Autodesk Inventor part; units mm, degrees
ref_plane "YZ Plane" through (0, 0, 0) normal (1, 0, 0) x (0, 1, 0)
ref_plane "XZ Plane" through (0, 0, 0) normal (0, 1, 0) x (-1, 0, 0)
ref_plane "XY Plane" through (0, 0, 0) normal (0, 0, 1) x (1, 0, 0)
sketch "Sketch2" plane through (0, 0, 0) normal (0, 0, 1) x (1, 0, 0)
  line L0 (-20, -20) -> (20, -20)
  line L1 (20, -20) -> (20, 20)
  line L2 (20, 20) -> (-20, 20)
  line L3 (-20, 20) -> (-20, -20)
  line L4 (-20, -20) -> (20, 20) construction
  line L5 (20, -20) -> (-20, 20) construction
  line L6 (-10, -10) -> (10, -10) construction
  line L7 (10, -10) -> (10, 10) construction
  line L8 (10, 10) -> (-10, 10) construction
  line L9 (-10, 10) -> (-10, -10) construction
  line L10 (-10, -10) -> (10, 10) construction
  line L11 (10, -10) -> (-10, 10) construction
  point P0 (0, 0)
  dimension "d0" = 40
  dimension "d1" = 40
  dimension "d2" = 20
  dimension "d3" = 20
extrude "Extrusion1" add sketch "Sketch2" along normal blind 5
hole "Hole1" at (-10, 10, 0) at (10, 10, 0) at (10, -10, 0) at (-10, -10, 0) direction (0, 0, 1) diameter 5.5 end through all
fillet "Fillet1" radius 2 4 edges at (20, 20, 2.5) (-20, 20, 2.5) (-20, -20, 2.5) (20, -20, 2.5)
properties part number "4040Square"
Input: part model. Units: mm. Frame: model coordinates. Give positions to 0.01 mm unless a question says otherwise; leave off trailing zeros. Loops run counter-clockwise (first coordinate to the right, second up) from the corner with the lowest first, then second, coordinate; pieces in that order, holes last. Notation, with made-up numbers: (55.5, 12) -> (94.5, 12) arc R23 cw to (94.5, 30) -> close; hole circle Ø11 at (-29.5, -19). An arc over 180 degrees is marked (long way). Use a Markdown table: item, result.
Q1. Pull-direction query (X, two-part tool) for faces 1 (the flat face through (0, 0, 5)), 2 (the cylindrical face through (-19.43, -19.4, 2.54)), 3 (the cylindrical face through (11.05, -7.46, 2.54)), 4 (the cylindrical face through (19.43, 19.4, 2.54)); classes: pulls with the +X half, pulls with the -X half, needs draft (parallel to the pull), parting line crosses it, or undercut.
Entries:
| item | result |
|---|---|
| face 1 | needs draft |
| face 2 | pulls with the -X half |
| face 3 | undercut |
| face 4 | pulls with the +X half |
Q2. Ray query, probe 1 along Y at (x, z) = (-10, 1.35); probe 2 along Y at (x, z) = (-11, 3.7); probe 3 along X at (y, z) = (8.5, 0.85). Return the intervals inside material, ascending. Write a range as from..to.
Entries:
| item | result |
|---|---|
| probe 1 | y = -20..-12.75, -7.25..7.25, 12.75..20 |
| probe 2 | y = -20..-12.56, -7.44..7.44, 12.56..20 |
| probe 3 | x = -20..-12.3, -7.7..7.7, 12.3..20 |
Q3. Section query A-A, the plane x = 10. Return the cut outline in (y, z).
Entries:
| item | result |
|---|---|
| outline | (-20, 0) -> (-12.75, 0) -> (-12.75, 5) -> (-20, 5) -> close; (-7.25, 0) -> (7.25, 0) -> (7.25, 5) -> (-7.25, 5) -> close; (12.75, 0) -> (20, 0) -> (20, 5) -> (12.75, 5) -> close |
Q4. First-contact query: P1, Ø5, axis at x = 10, y = 10, coming from the +Z side. Flat tip, straight axial feed; report the tip coordinate or a pass-through.
Entries:
| item | result |
|---|---|
| P1 | passes through |
Q5. Section query C-C, the plane z = 2.75. Return the cut outline in (x, y), plus the area to 3 significant figures.
Entries:
| item | result |
|---|---|
| outline | (-20, -18) arc R2 ccw to (-18, -20) -> (18, -20) arc R2 ccw to (20, -18) -> (20, 18) arc R2 ccw to (18, 20) -> (-18, 20) arc R2 ccw to (-20, 18) -> close; hole circle Ø5.5 at (-10, -10); hole circle Ø5.5 at (-10, 10); hole circle Ø5.5 at (10, -10); hole circle Ø5.5 at (10, 10) |
| area | 1,500 mm² |
